from build123d import *

# Parameters (mm, degrees)
SKETCH_1_R          = 12.5
EXTRUDE_1_DEPTH     = 4
SKETCH_2_R          = 12.5
SKETCH_2_R_2        = 10
EXTRUDE_2_DEPTH     = 3.5
SKETCH_3_R          = 1.5
CUT_EXTRUDE_1_DEPTH = 53.08166664
EXTRUDE_3_DEPTH     = 25
SKETCH_5_W          = 7
SKETCH_5_H          = 5
CUT_EXTRUDE_2_DEPTH = 57.621550668
SKETCH_6_W          = 7
SKETCH_6_H          = 5
CUT_EXTRUDE_3_DEPTH = 52.780787943
SKETCH_7_R          = 10
SKETCH_7_R_2        = 1.5
EXTRUDE_4_DEPTH     = 1


with BuildPart() as part:
    # 草图1 → 凸台-拉伸1 (new body)
    with BuildSketch(Plane(origin=(0, 0, 0), x_dir=(1, 0, 0), z_dir=(0, 1, 0))):
        Circle(SKETCH_1_R)
        with BuildLine():
            Line((50, 12.5), (0, 12.5))
            ThreePointArc((0, 12.5), (8.838834765, 8.838834765), (12.5, 0))
            ThreePointArc((12.5, 0), (8.838834765, -8.838834765), (0, -12.5))
            Line((0, -12.5), (50, -12.5))
            Line((50, -12.5), (50, 12.5))
        make_face()
    extrude(amount=EXTRUDE_1_DEPTH)

    # 草图2 → 凸台-拉伸2 (add)
    with BuildSketch(Plane(origin=(0, 4, 0), x_dir=(1, 0, 0), z_dir=(0, 1, 0))):
        with Locations(Location((0, 0, 0), (0, 0, 270))):
            Circle(SKETCH_2_R)
        with Locations(Location((0, 0, 0), (0, 0, 270))):
            Circle(SKETCH_2_R_2, mode=Mode.SUBTRACT)
    extrude(amount=EXTRUDE_2_DEPTH)

    # 草图3 → 切除-拉伸1 (cut, through all)
    with BuildSketch(Plane.XZ):
        with Locations(Location((0, 0, 0), (0, 0, 270))):
            Circle(SKETCH_3_R)
        with Locations(Location((0, 7, 0), (0, 0, 270))):
            Circle(SKETCH_3_R)
        with Locations(Location((7, 0, 0), (0, 0, 270))):
            Circle(SKETCH_3_R)
        with Locations(Location((0, -7, 0), (0, 0, 270))):
            Circle(SKETCH_3_R)
        with Locations(Location((-7, 0, 0), (0, 0, 270))):
            Circle(SKETCH_3_R)
        with Locations(Location((40, 0, 0), (0, 0, 270))):
            Circle(SKETCH_3_R)
    extrude(amount=-CUT_EXTRUDE_1_DEPTH, mode=Mode.SUBTRACT)

    # 草图4 → 凸台-拉伸3 (add)
    with BuildSketch(Plane.XY.offset(12.5)):
        Polygon((50, 4), (47, 9), (33, 9), (30, 4), align=None)
    extrude(amount=-EXTRUDE_3_DEPTH)

    # 草图5 → 切除-拉伸2 (cut, through all)
    with BuildSketch(Plane.XY.offset(12.5)):
        with Locations((40, 6.5)):
            Rectangle(SKETCH_5_W, SKETCH_5_H)
    extrude(amount=-CUT_EXTRUDE_2_DEPTH, mode=Mode.SUBTRACT)

    # 草图6 → 切除-拉伸3 (cut, through all)
    with BuildSketch(Plane(origin=(0, 4, 0), x_dir=(1, 0, 0), z_dir=(0, 1, 0))):
        with Locations((40, -10)):
            Rectangle(SKETCH_6_W, SKETCH_6_H)
        with Locations((40, 10)):
            Rectangle(SKETCH_6_W, SKETCH_6_H)
    extrude(amount=-CUT_EXTRUDE_3_DEPTH, mode=Mode.SUBTRACT)

    # 草图7 → 凸台-拉伸4 (add)
    with BuildSketch(Plane(origin=(0, 4, 0), x_dir=(1, 0, 0), z_dir=(0, 1, 0))):
        with Locations(Location((0, 0, 0), (0, 0, 270))):
            Circle(SKETCH_7_R)
        with Locations(Location((0, 0, 0), (0, 0, 90))):
            Circle(SKETCH_7_R_2, mode=Mode.SUBTRACT)
        with Locations(Location((0, 7, 0), (0, 0, 90))):
            Circle(SKETCH_7_R_2, mode=Mode.SUBTRACT)
        with Locations(Location((7, 0, 0), (0, 0, 90))):
            Circle(SKETCH_7_R_2, mode=Mode.SUBTRACT)
        with Locations(Location((0, -7, 0), (0, 0, 90))):
            Circle(SKETCH_7_R_2, mode=Mode.SUBTRACT)
        with Locations(Location((-7, 0, 0), (0, 0, 90))):
            Circle(SKETCH_7_R_2, mode=Mode.SUBTRACT)
    extrude(amount=EXTRUDE_4_DEPTH)


solid = part.part
Work out the finished part from the listing and answer in its coordinate system (mm). A direction names the side the tool comes from. Round coordinates to 2 decimals unless told otherwise and drop trailing zeros. Write each loop counter-clockwise with the first axis right and the second up, starting at its lowest first coordinate (ties: lowest second). Pieces come first, ordered by that corner, then holes. Notation, with made-up numbers: (71.25, 64) - (128.25, 64) arc R18 ccw to (128.25, 79) - close; hole circle Ø4 at (4, 83). An arc over 180 degrees is marked (long way). Answer in a Markdown table with one row per item. Add a question column.
1. Find the intervals of material crossed by line 1 along X through (y, z) = (3.1, 0); line 2 along Z through (x, y) = (-1, 2.75); line 3 along X through (y, z) = (6.25, -0.5), in increasing order. Write a range as from..to.
2. For faces 1 (the flat face through (43.5, 5, 0)), 2 (the flat face through (42, 4, 0)), 3 (the flat face through (40, 2, 7.5)), determine the directions among +Z, -Z, +X, -X, +Y, -Y from which every point of the face is accessible in a straight line to the end or side of a thin tool.
3. The mould has two halves that part along Z. Classify faces 4 (the flat face through (45, 9, 0)), 5 (the cylindrical face through (-0.07, 2.46, 8.5)), 6 (the flat face through (40, 2, -7.5)): +Z half, -Z half, draft (parallel to the pull), parting line (faces both ways), or undercut.
4. A cutting plane is placed at D-D, the plane x = -7. Determine the outline of the cut face in (y, z).
5. A cutting plane is placed at A-A, the plane y = 6.25. Determine the outline of the cut face in (x, z).
6. A cutting plane is placed at B-B, the plane z = 0. Count the separate pieces of the cut face and the enclosed holes in it, and give its area (4 significant figures).
7. Given pin 1 (1.5 mm diameter, centred on x = -3, y = 1.5, fed in from +Z); pin 2 (4 mm diameter, centred on x = 0, z = 7, fed in from +Y); pin 3 (7.5 mm diameter, centred on x = -6, z = 2, fed in from +Y), each flat-ended and moving along its own axis, determine where each tip first touches the part or whether it passes through.
8. A cutting plane is placed at C-C, the plane y = 1.5. Determine the outline of the cut face in (x, z).
Worked out:
| question | item | result |
|---|---|---|
| 1 | line 1 | -12.5..-8.5, -5.5..-1.5, 1.5..5.5, 8.5..38.5, 41.5..50 |
| 1 | line 2 | -12.46..-8.12, -5.88..-1.12, 1.12..5.88, 8.12..12.46 |
| 1 | line 3 | -12.49..-9.99, 9.99..12.49, 31.35..36.5, 43.5..48.65 |
| 2 | face 1 | +Y |
| 2 | face 2 | +Z, -Z, +Y |
| 2 | face 3 | +Z, +Y, -Y |
| 3 | face 4 | draft |
| 3 | face 5 | undercut |
| 3 | face 6 | -Z half |
| 4 | outline | (0, -10.36) - (7.5, -10.36) - (7.5, -7.14) - (5, -7.14) - (5, -1.5) - (0, -1.5) - close; (0, 1.5) - (5, 1.5) - (5, 7.14) - (7.5, 7.14) - (7.5, 10.36) - (0, 10.36) - close |
| 5 | outline | circle Ø25 at (0, 0); (31.35, -12.5) - (36.5, -12.5) - (36.5, 12.5) - (31.35, 12.5) - close; (43.5, -12.5) - (48.65, -12.5) - (48.65, 12.5) - (43.5, 12.5) - close; hole circle Ø20 at (0, 0) |
| 6 | separate pieces | 5 |
| 6 | enclosed holes | 0 |
| 6 | area | 280.5 mm^2 |
| 7 | pin 1 | z = 12.3 |
| 7 | pin 2 | y = 5 |
| 7 | pin 3 | y = 7.5 |
| 8 | outline | (0, -12.5) - (36.5, -12.5) - (36.5, -7.5) - (43.5, -7.5) - (43.5, -12.5) - (50, -12.5) - (50, 12.5) - (43.5, 12.5) - (43.5, 7.5) - (36.5, 7.5) - (36.5, 12.5) - (0, 12.5) arc R12.5 ccw to start; hole circle Ø3 at (-7, 0); hole circle Ø3 at (0, -7); hole circle Ø3 at (0, 0); hole circle Ø3 at (0, 7); hole circle Ø3 at (7, 0); hole circle Ø3 at (40, 0) |
